Read the model definition and answer for the solid it produces. Units are mm, in the model's axes. Coordinates: 2 decimals unless noted, no trailing zeros. Write each loop counter-clockwise with the first axis right and the second up, starting at its lowest first coordinate (ties: lowest second). Pieces come first, ordered by that corner, then holes. Notation, with made-up numbers: (21.5, 76) -> (45.5, 76) arc R26 cw to (45.5, 111) -> close; hole circle Ø11 at (-12, 9). An arc over 180 degrees is marked (long way). Answer in a Markdown table with one row per item. Add a question column.
Item 1: Section A-A on x = 0 is taken. Write down the section's boundary in (y, z), then the cut area to 3 significant figures.
Item 2: Section B-B on y = 11 is taken. Write down the section's boundary in (x, z), then the cut area to 3 significant figures.
Item 3: Straight lines are drawn through the part: line 1 (Y direction, x = 0, z = 0.3); line 2 (X direction, y = -10, z = 0.2); line 3 (X direction, y = 2.5, z = 0.4). For each, find the intervals that lie inside material, in ascending order. Write a range as from..to.
Item 4: Section D-D on y = 0 is taken. Write down the section's boundary in (x, z).
Item 5: Given pin 1 Ø7 at (x, y) = (0, 0) entering from -Z, flat-ended and moving along its own axis, determine where the tip first touches the part or whether it passes through.
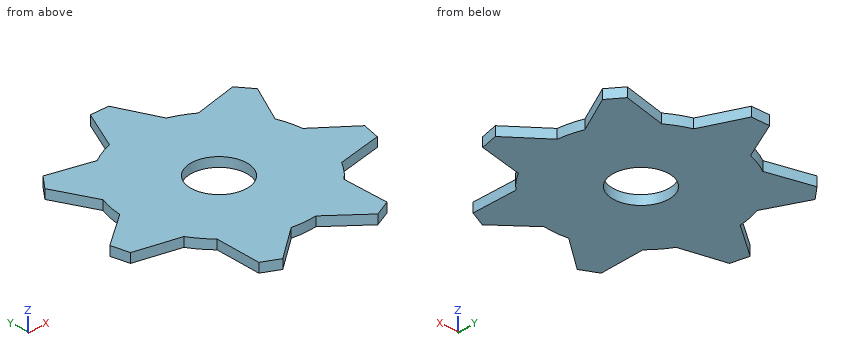
```python
from build123d import *

# Parameters (mm, degrees)
SKETCH1_R           = 12.7
BOSS_EXTRUDE1_DEPTH = 1.27
BOSS_EXTRUDE2_DEPTH = 1.27
CIRPATTERN1_COUNT   = 7
SKETCH4_R           = 3.81
CUT_EXTRUDE1_DEPTH  = 1.27


with BuildPart() as part:
    # Sketch1 → Boss-Extrude1 (new body)
    with BuildSketch(Plane.XY):
        Circle(SKETCH1_R)
    extrude(amount=BOSS_EXTRUDE1_DEPTH)

    # Sketch3 → Boss-Extrude2 (add)
    with BuildSketch(Plane.XY.offset(1.27)):
        Polygon((0, 17.78), (-1.27, 17.78), (-3.929437707, 12.076817433), (3.929437707, 12.076817433), (1.27, 17.78), align=None)
    boss_extrude2 = extrude(amount=-BOSS_EXTRUDE2_DEPTH)

    # CirPattern1: Boss-Extrude2 ×7 about axis
    cirpattern1_axis = Axis((0, 0, 0), (0, 0, 1))
    for i in range(1, CIRPATTERN1_COUNT):
        add(boss_extrude2.rotate(cirpattern1_axis, i * 360 / CIRPATTERN1_COUNT))

    # Sketch4 → Cut-Extrude1 (cut)
    with BuildSketch(Plane(origin=(0, 0, 0), x_dir=(-1, 0, 0), z_dir=(0, 0, -1))):
        Circle(SKETCH4_R)
    extrude(amount=-CUT_EXTRUDE1_DEPTH, mode=Mode.SUBTRACT)


solid = part.part
```
Results below:
| question | item | result |
|---|---|---|
| 1 | outline | (-12.7, 0) -> (-3.81, 0) -> (-3.81, 1.27) -> (-12.7, 1.27) -> close; (3.81, 0) -> (17.78, 0) -> (17.78, 1.27) -> (3.81, 1.27) -> close |
| 1 | area | 29.0 mm2 |
| 2 | outline | (-13.97, 0) -> (-8.64, 0) -> (-8.64, 1.27) -> (-13.97, 1.27) -> close; (-6.35, 0) -> (6.35, 0) -> (6.35, 1.27) -> (-6.35, 1.27) -> close; (8.64, 0) -> (13.97, 0) -> (13.97, 1.27) -> (8.64, 1.27) -> close |
| 2 | area | 29.7 mm2 |
| 3 | line 1 | y = -12.7..-3.81, 3.81..17.78 |
| 3 | line 2 | x = -8.79..8.79 |
| 3 | line 3 | x = -12.45..-2.88, 2.88..12.45 |
| 4 | outline | (-14.12, 0) -> (-3.81, 0) -> (-3.81, 1.27) -> (-14.12, 1.27) -> close; (3.81, 0) -> (14.12, 0) -> (14.12, 1.27) -> (3.81, 1.27) -> close |
| 5 | pin 1 | passes through |
